For this review, use the dimensioned drawing (mm, ordinates from the lowest corner) and the shaded views. A direction names the side the tool comes from. Round coordinates to 2 decimals unless told otherwise and drop trailing zeros. Loops run counter-clockwise (first coordinate to the right, second up) from the corner with the lowest first, then second, coordinate; pieces in that order, holes last. Notation, with made-up numbers: M -3,53 L 11,53 A19 cw 11,85 Z; hole C -29,62.5 d4. An arc over 180 degrees is marked long. One line per item, written item: value. Start each with the question number.
Item 1: We need section B-B (x = 12.5). Write out the cut boundary in (y, z), then the cut area to 3 significant figures.
Item 2: For the marked faces 3 and 4, list the 3-axis set-ups (+Z, -Z, +X, -X, +Y, -Y) from which the entire face can be reached by the end or side of a thin tool; tool diameter is ignored.
Item 3: Mouldability with a two-part tool opening along X and no side actions: class the marked faces 1 and 2 as released by +X, released by -X, zero draft, split by the parting line, or undercut.
Item 4: Clearance check with flat-ended pins moving along their axes: pin 1 (4 mm diameter, centred on x = 51.5, y = 8, fed in from -Z); pin 2 (0.6 mm diameter, centred on x = 0.5, z = 2.5, fed in from +Y); pin 3 (2 mm diameter, centred on y = 8, z = 3, fed in from +X); pin 4 (1.8 mm diameter, centred on y = 9, z = 4, fed in from +X). State where each tip first meets the part, or that it passes through.
Item 5: For line 1 along Y through (x, z) = (51.5, 4.9); line 2 along X through (y, z) = (2.5, 3.5); line 3 along Z through (x, y) = (62.5, 8), list the stretches that pass through material, from the lowest coordinate up.
Item 6: We need section C-C (y = 10). Write out the cut boundary in (x, z), then the cut area to 3 significant figures.
Item 7: We need section A-A (z = 0.85). Write out the cut boundary in (x, y).
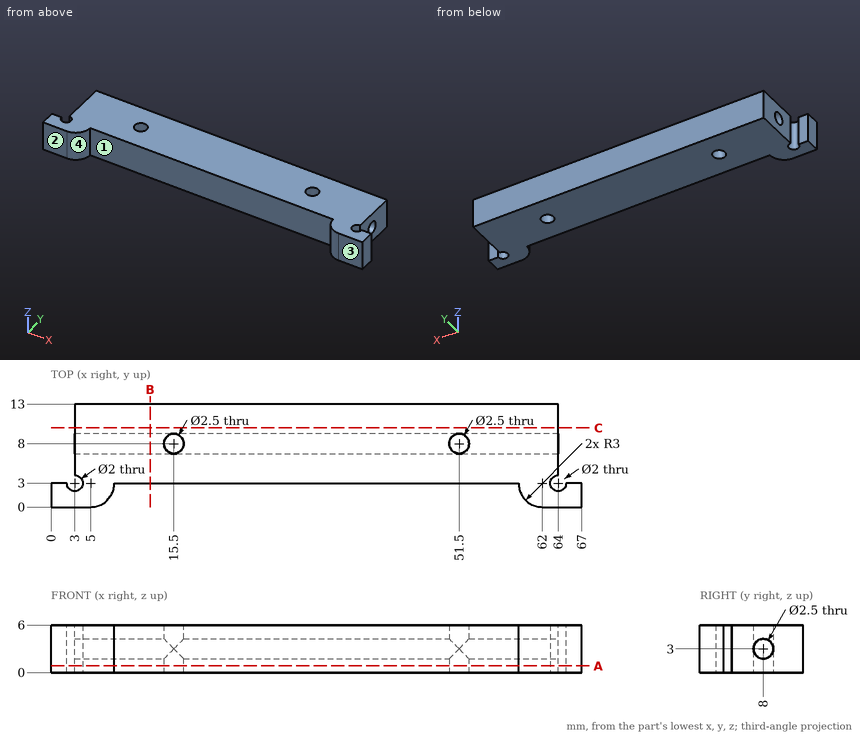
A:
1. outline: M 3,0 L 13,0 L 13,6 L 3,6 Z; hole C 8,3 d2.5
1. area: 55.1 mm2
2. face 3: +Z, -Z, +X, -X, -Y
2. face 4: +Z, -Z, -Y
3. face 1: undercut
3. face 2: zero draft
4. pin 1: z = 0
4. pin 2: y = 3
4. pin 3: through
4. pin 4: x = 64
5. line 1: 3 to 6.75, 9.25 to 13
5. line 2: 0 to 2.13, 3.87 to 7.96, 59.04 to 63.13, 64.87 to 67
5. line 3: 0 to 1.75, 4.25 to 6
6. outline: M 3,0 L 64,0 L 64,6 L 3,6 Z
6. area: 366 mm2
7. outline: M 0,0 L 5,0 A3 ccw 8,3 L 59,3 A3 ccw 62,0 L 67,0 L 67,3 L 65,3 A1 cw long 64,4 L 64,13 L 3,13 L 3,4 A1 cw long 2,3 L 0,3 Z; hole C 15.5,8 d2.5; hole C 51.5,8 d2.5
